CAD build for the part. Positions are in the model's coordinates, mm. Face numbers are marked on the shaded views. Coordinates: 2 decimals unless noted, no trailing zeros. Write each loop counter-clockwise with the first axis right and the second up, starting at its lowest first coordinate (ties: lowest second). Pieces come first, ordered by that corner, then holes. Notation, with made-up numbers: (68.5, 32) -> (119.5, 32) arc R11 cw to (119.5, 42) -> close; hole circle Ø1 at (3.5, 64). An arc over 180 degrees is marked (long way). Answer as CSV lines item,"result".
```python
from build123d import *

# Parameters (mm, degrees)
F0_R     = 2.54
F1_DEPTH = 1.5875


with BuildPart() as f1:
    # F0 (on Right) → F1 (new body)
    with BuildSketch(Plane.YZ):
        with BuildLine():
            Line((10.213834, 5.08), (-12.011166, 5.08))
            Line((-12.011166, 5.08), (-12.011166, -5.08))
            Line((-12.011166, -5.08), (10.213834, -5.08))
            ThreePointArc((10.213834, -5.08), (5.133834, 0), (10.213834, 5.08))
        make_face()
        with BuildLine():
            ThreePointArc((-8.836166, -3.33375), (-9.629916, -2.54), (-8.836166, -1.74625))
            Line((-8.836166, -1.74625), (1.323834, -1.74625))
            ThreePointArc((1.323834, -1.74625), (1.8851, -1.978734), (2.117584, -2.54))
            ThreePointArc((2.117584, -2.54), (1.8851, -3.101266), (1.323834, -3.33375))
            Line((1.323834, -3.33375), (-8.836166, -3.33375))
        make_face(mode=Mode.SUBTRACT)
        with BuildLine():
            ThreePointArc((-8.836166, 1.74625), (-9.629916, 2.54), (-8.836166, 3.33375))
            Line((-8.836166, 3.33375), (1.323834, 3.33375))
            ThreePointArc((1.323834, 3.33375), (1.8851, 3.101266), (2.117584, 2.54))
            ThreePointArc((2.117584, 2.54), (1.8851, 1.978734), (1.323834, 1.74625))
            Line((1.323834, 1.74625), (-8.836166, 1.74625))
        make_face(mode=Mode.SUBTRACT)
        with BuildLine():
            ThreePointArc((15.293834, 0), (13.805936, 3.592102), (10.213834, 5.08))
            ThreePointArc((10.213834, 5.08), (5.133834, 0), (10.213834, -5.08))
            ThreePointArc((10.213834, -5.08), (13.805936, -3.592102), (15.293834, 0))
        make_face()
        with Locations((10.213834, 0)):
            Circle(F0_R, mode=Mode.SUBTRACT)
    extrude(amount=F1_DEPTH)


solid = f1.part
```
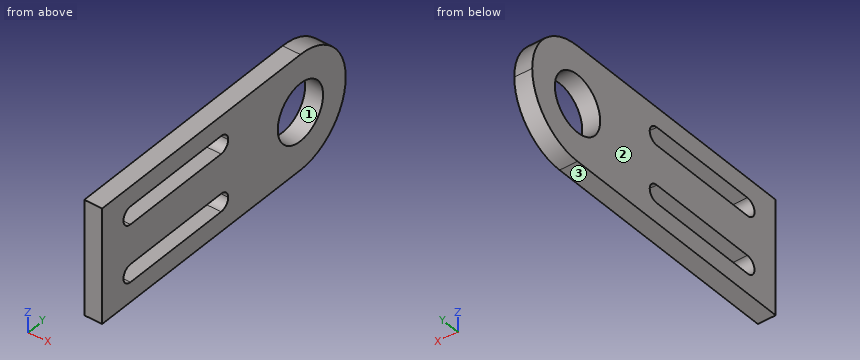
Item 1: Saw through at C-C on z = 0.5. Give the cut face in (x, y), and give its area (3 significant figures).
Answer below:
outline,"(0, -12.01) -> (1.59, -12.01) -> (1.59, 7.72) -> (0, 7.72) -> close; (0, 12.7) -> (1.59, 12.7) -> (1.59, 15.27) -> (0, 15.27) -> close"
area,"35.4 mm2"
Item 2: Saw through at B-B on x = 1.05. Give the cut face in (y, z), and give its area (3 significant figures).
Answer below:
outline,"(-12.01, -5.08) -> (10.21, -5.08) arc R5.08 ccw to (15.29, 0) arc R5.08 ccw to (10.21, 5.08) -> (-12.01, 5.08) -> close; hole (-8.84, -3.33) -> (1.32, -3.33) arc R0.79 ccw to (1.32, -1.75) -> (-8.84, -1.75) arc R0.79 ccw to start; hole (-8.84, 1.75) -> (1.32, 1.75) arc R0.79 ccw to (1.32, 3.33) -> (-8.84, 3.33) arc R0.79 ccw to start; hole circle Ø5.08 at (10.21, 0)"
area,"210 mm2"
Item 3: Two-plate mould, pull along Z, no slides. Class the marked faces 1, 2 and 3: pulls with the +Z half, pulls with the -Z half, needs draft (parallel to the pull), parting line crosses it, or undercut.
Answer below:
face 1,"undercut"
face 2,"needs draft"
face 3,"pulls with the -Z half"
Item 4: Wall check: line 1 (Z direction, x = 0.1, y = -1.5); line 2 (Y direction, x = 0.65, z = 1); line 3 (Y direction, x = 0.45, z = -0.25). Give the ranges that are in metal, low to high. Write a range as from..to.
Answer below:
line 1,"z = -5.08..-3.33, -1.75..1.75, 3.33..5.08"
line 2,"y = -12.01..7.88, 12.55..15.19"
line 3,"y = -12.01..7.69, 12.74..15.29"
Item 5: Saw through at D-D on z = 2.25. Give the cut face in (x, y).
Answer below:
outline,"(0, -12.01) -> (1.59, -12.01) -> (1.59, -9.58) -> (0, -9.58) -> close; (0, 2.06) -> (1.59, 2.06) -> (1.59, 9.04) -> (0, 9.04) -> close; (0, 11.39) -> (1.59, 11.39) -> (1.59, 14.77) -> (0, 14.77) -> close"
Item 6: Saw through at A-A on y = -1. Give the cut face in (x, z).
Answer below:
outline,"(0, -5.08) -> (1.59, -5.08) -> (1.59, -3.33) -> (0, -3.33) -> close; (0, -1.75) -> (1.59, -1.75) -> (1.59, 1.75) -> (0, 1.75) -> close; (0, 3.33) -> (1.59, 3.33) -> (1.59, 5.08) -> (0, 5.08) -> close"
